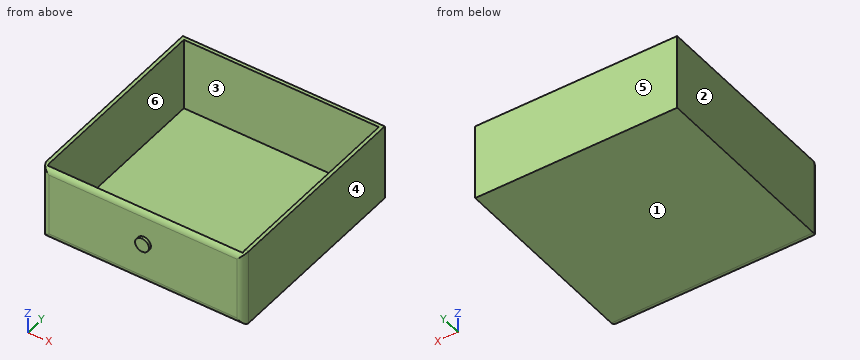
```python
from build123d import *

# Parameters (mm, degrees)
F0_W        = 145
F0_H        = 145
F1_DEPTH    = 55
F2_T        = -2.5
F3_T1_DEPTH = 80
F3_T3_DEPTH = 170
F5_DEPTH    = 2


# Not quite as in the source:
# - a fillet or chamfer that OpenCascade refuses, or shapes differently, is made with other operations: its cross-section is extruded or revolved along the edge and cut away or added


with BuildPart() as f1:
    # F0 (on Top) → F1 (new body)
    with BuildSketch(Plane.XY):
        with Locations((-0.7837880796, -0.1337006688)):
            Rectangle(F0_W, F0_H)
    extrude(amount=F1_DEPTH)

    # F2
    f2_openings = [f1.faces().sort_by_distance(p)[0] for p in [
        (-0.783788, -0.133701, 55),
    ]]
    offset(amount=F2_T, openings=f2_openings)

    # F3: fillet of radius 5 on 4 edges, made by hand

    # F3_s2 → F3_t1 (cut)
    with BuildSketch(Plane.XY.offset(-12.5)):
        with BuildLine():
            ThreePointArc((-73.2837880796, -67.6337006688), (-71.8193219856, -71.1692345747), (-68.2837880796, -72.6337006688))
            Line((-68.2837880796, -72.6337006688), (-73.2837880796, -72.6337006688))
            Line((-73.2837880796, -72.6337006688), (-73.2837880796, -67.6337006688))
        make_face()
        with BuildLine():
            ThreePointArc((66.7162119204, -72.6337006688), (70.2517458263, -71.1692345747), (71.7162119204, -67.6337006688))
            Line((71.7162119204, -67.6337006688), (71.7162119204, -72.6337006688))
            Line((71.7162119204, -72.6337006688), (66.7162119204, -72.6337006688))
        make_face()
    extrude(amount=F3_T1_DEPTH, mode=Mode.SUBTRACT)

    # F3_s4 → F3_t3 (cut)
    with BuildSketch(Plane.YZ.offset(-85.7837880796)):
        with BuildLine():
            ThreePointArc((-72.6337006688, 5), (-71.1692345747, 1.4644660941), (-67.6337006688, 0))
            Line((-67.6337006688, 0), (-72.6337006688, 0))
            Line((-72.6337006688, 0), (-72.6337006688, 5))
        make_face()
        with BuildLine():
            ThreePointArc((-72.6337006688, 50), (-71.1692345747, 53.5355339059), (-67.6337006688, 55))
            Line((-67.6337006688, 55), (-72.6337006688, 55))
            Line((-72.6337006688, 55), (-72.6337006688, 50))
        make_face()
    extrude(amount=F3_T3_DEPTH, mode=Mode.SUBTRACT)

    # F4 (on face) → F5 (join)
    with BuildSketch(Plane.XZ.offset(72.6337006688)):
        with BuildLine():
            ThreePointArc((0, 25.2702692018), (3.5355339059, 26.7347352958), (5, 30.2702692018))
            ThreePointArc((5, 30.2702692018), (3.5355339059, 33.8058031077), (0, 35.2702692018))
            Line((0, 35.2702692018), (0, 25.2702692018))
        make_face()
        with BuildLine():
            Line((0, 25.2702692018), (0, 35.2702692018))
            ThreePointArc((0, 35.2702692018), (-5, 30.2702692018), (0, 25.2702692018))
        make_face()
    extrude(amount=F5_DEPTH)


solid = f1.part
```
Input: part model. Units: mm. Frame: model coordinates. Face numbers are marked on the shaded views. A direction names the side the tool comes from. Give positions to 0.01 mm unless a question says otherwise; leave off trailing zeros. Order: outer loops, then holes, each group sorted by start corner. A loop starts at its lowest first (then second) coordinate and runs counter-clockwise, first axis right, second up.
1. Cut plane B-B (z = 18). Return loops of the section in (x, y), and give its area (3 significant figures).
Computed:
outline: (-73.28, -67.63) arc R5 ccw to (-68.28, -72.63) - (66.72, -72.63) arc R5 ccw to (71.72, -67.63) - (71.72, 72.37) - (-73.28, 72.37) - close; hole (-70.78, -70.13) - (69.22, -70.13) - (69.22, 69.87) - (-70.78, 69.87) - close
area: 1,410 mm2
2. Cut plane C-C (y = 43.5). Return loops of the section in (x, z).
Computed:
outline: (-73.28, 0) - (71.72, 0) - (71.72, 55) - (69.22, 55) - (69.22, 2.5) - (-70.78, 2.5) - (-70.78, 55) - (-73.28, 55) - close
3. Set-up query: the marked faces 5 and 6. Return all of +Z, -Z, +X, -X, +Y, -Y with unobstructed straight access to the full face (end or side cutting, diameter ignored); none if empty.
Computed:
face 5: +Z, -Z, +X, -X, +Y
face 6: +Z
4. Line query: probe 1 along Y at (x, z) = (-66.5, 50.5); probe 2 along X at (y, z) = (61.5, 4.5); probe 3 along Z at (x, y) = (6, -21.5). Output: solid intervals per line, ascending.
Computed:
probe 1: y = -72.61 to -70.13, 69.87 to 72.37
probe 2: x = -73.28 to -70.78, 69.22 to 71.72
probe 3: z = 0 to 2.5
5. Draft query along X for the marked faces 1, 2, 3 and 4. Return one class per face: released by +X, released by -X, zero draft, split by the parting line, or undercut.
Computed:
face 1: zero draft
face 2: released by -X
face 3: undercut
face 4: released by +X
6. Cut plane A-A (x = -8.5). Return loops of the section in (y, z), and give its area (3 significant figures).
Computed:
outline: (-72.63, 5) arc R5 ccw to (-67.63, 0) - (72.37, 0) - (72.37, 55) - (69.87, 55) - (69.87, 2.5) - (-70.13, 2.5) - (-70.13, 54.33) arc R5 ccw to (-72.63, 50) - close
area: 615 mm2
7. Pin query (flat end, axial travel): pin 1 Ø1 at (x, y) = (-1, 39.5) entering from -Z; pin 2 Ø1.5 at (x, z) = (31.5, 12) entering from -Y; pin 3 Ø10 at (x, y) = (-15.5, 12.5) entering from +Z. Return the tip coordinate at first contact, or that it passes through.
Computed:
pin 1: stops at z = 0
pin 2: stops at y = -72.63
pin 3: stops at z = 2.5
